The listing builds one solid part. Answer for the finished solid, in the listing's coordinates (mm). A direction names the side the tool comes from. Give positions to 0.01 mm unless a question says otherwise; leave off trailing zeros. Loops run counter-clockwise (first coordinate to the right, second up) from the corner with the lowest first, then second, coordinate; pieces in that order, holes last.
Item 1: Section C-C, the plane z = 113.5 is taken. Give the vertices of the cut face in (x, y).
Item 2: A tool of negligible diameter and unlimited length cuts with its end or side. For faces 5 (the face through (-74.674, -14, 64)), 6 (the face through (-125, 48, 50.8)), 7 (the face through (-0.8, -3.2, 64.4)), from which of +Z, -Z, +X, -X, +Y, -Y can it reach the whole face along a straight path? Write none if from no direction.
Item 3: Each of these flat-tipped pins is pushed along its axis until it touches: pin 1 Ø6 at (x, y) = (10.5, 15.5) entering from +Z; pin 2 Ø8 at (y, z) = (60, 35.5) entering from -X; pin 3 Ø2 at (x, z) = (-116.5, 57) entering from -Y. Where does it stop, or does it pass through?
Item 4: Section D-D, the plane y = 28 is taken. Give the vertices of the cut face in (x, z).
Item 5: Section B-B, the plane x = -92 is taken. Give the vertices of the cut face in (y, z), and give its area (3 significant figures).
Item 6: The mould has two halves that part along Y. Classify faces 1 (the face through (-55.417, 34.887, 89.269)), 2 (the face through (-105, 8.901, 79)), 3 (the face through (28.746, 50.696, 64.389)), 4 (the face through (-19, 26, 0)): pulls with the +Y half, pulls with the -Y half, needs draft (parallel to the pull), parting line crosses it, or undercut.
Item 7: Section A-A, the plane z = 91 is taken. Give the vertices of the cut face in (x, y), and give its area (3 significant figures).
Item 8: Consider line 1 along Z through (x, y) = (-29, 47); line 2 along Y through (x, z) = (-2, 90); line 3 along Y through (x, z) = (12, 91). Determine where each line is inside the solid, lowest interval first.
from build123d import *

# Parameters (mm, degrees)
F0_W      = 215.9
F0_H      = 120.65
F1_DEPTH  = 127
F2_W      = 76.2
F2_H      = 44.45
F3_DEPTH  = 25.4
F3_FACE_W = 76.2
F3_FACE_H = 44.45
F4_DEPTH  = 101.601
F6_DEPTH  = 127.001
F7_W      = 50.8
F7_H      = 50.8
F8_DEPTH  = 120.651
F9_R      = 12.7
F10_DEPTH = 215.901
F12_R     = 12.7
F13_DEPTH = 127.001


with BuildPart() as f1:
    # F0 (on Top) → F1 (new body)
    with BuildSketch(Plane.XY):
        with Locations((-42.923508, 24.775881)):
            Rectangle(F0_W, F0_H)
    extrude(amount=F1_DEPTH)

    # F2 (on face) → F3 (cut)
    with BuildSketch(Plane.XY.offset(127)):
        with Locations((-112.773508, -13.324119)):
            Rectangle(F2_W, F2_H)
    extrude(amount=-F3_DEPTH, mode=Mode.SUBTRACT)

    # F3_face (on face) → F4 (cut, through all)
    with BuildSketch(Plane(origin=(-112.773508, -13.324119, 101.6), x_dir=(1, 0, 0), z_dir=(0, 0, 1))):
        Rectangle(F3_FACE_W, F3_FACE_H)
    extrude(amount=-F4_DEPTH, mode=Mode.SUBTRACT)

    # F5 (on face) → F6 (cut, through all)
    with BuildSketch(Plane.XY.offset(127)):
        with BuildLine():
            ThreePointArc((-55.623508, 85.100881), (29.688925, 49.763314), (65.026492, -35.549119))
            Line((65.026492, -35.549119), (65.026492, 85.100881))
            Line((65.026492, 85.100881), (-55.623508, 85.100881))
        make_face()
    extrude(amount=-F6_DEPTH, mode=Mode.SUBTRACT)

    # F7 (on face) → F8 (cut, through all)
    with BuildSketch(Plane(origin=(0, 85.100881, 0), x_dir=(-1, 0, 0), z_dir=(0, 1, 0))):
        with Locations((125.473508, 25.4)):
            Rectangle(F7_W, F7_H)
    extrude(amount=-F8_DEPTH, mode=Mode.SUBTRACT)

    # F9 (on face) → F10 (cut, through all)
    with BuildSketch(Plane(origin=(-150.873508, 0, 0), x_dir=(0, -1, 0), z_dir=(-1, 0, 0))):
        with Locations((-47.000881, 85.454322)):
            Circle(F9_R)
    extrude(amount=-F10_DEPTH, mode=Mode.SUBTRACT)

    # F12 (on face) → F13 (cut, through all)
    with BuildSketch(Plane.XY.offset(127)):
        with Locations((1.959576, 9.196907)):
            Circle(F12_R)
    extrude(amount=-F13_DEPTH, mode=Mode.SUBTRACT)


solid = f1.part
Worked answers:
1. outline: (-150.87, 8.9) - (-74.67, 8.9) - (-74.67, -35.55) - (65.03, -35.55) arc R120.65 ccw to (-55.62, 85.1) - (-150.87, 85.1) - close; hole circle Ø25.4 at (1.96, 9.2)
2. face 5: +Z, -Z, -X, -Y
2. face 6: -Z, -X, +Y, -Y
2. face 7: +Z, -Z
3. pin 1: stops at z = 127
3. pin 2: stops at x = -100.07
3. pin 3: stops at y = 8.9
4. outline: (-150.87, 50.8) - (-100.07, 50.8) - (-100.07, 0) - (46.93, 0) - (46.93, 127) - (-150.87, 127) - close
5. outline: (8.9, 0) - (85.1, 0) - (85.1, 127) - (8.9, 127) - close; hole circle Ø25.4 at (47, 85.45)
5. area: 9,170 mm2
6. face 1: undercut
6. face 2: pulls with the -Y half
6. face 3: pulls with the +Y half
6. face 4: needs draft
7. outline: (-150.87, 8.9) - (-74.67, 8.9) - (-74.67, -35.55) - (65.03, -35.55) arc R120.65 ccw to (41.83, 35.58) - (-150.87, 35.58) - close; (-150.87, 58.43) - (20.04, 58.43) arc R120.65 ccw to (-55.62, 85.1) - (-150.87, 85.1) - close; hole circle Ø25.4 at (1.96, 9.2)
7. area: 14,900 mm2
8. line 1: z = 0 to 72.75, 98.15 to 127
8. line 2: y = -35.55 to -2.87, 21.26 to 35.14, 58.86 to 72.53
8. line 3: y = -35.55 to 1.42, 16.97 to 35.58, 58.43 to 64.37
